Verification items for the finished model (mm, model axes). Face numbers are marked on the shaded views. A direction names the side the tool comes from. Coordinates: 2 decimals unless noted, no trailing zeros. Write each loop counter-clockwise with the first axis right and the second up, starting at its lowest first coordinate (ties: lowest second). Pieces come first, ordered by that corner, then holes. Notation, with made-up numbers: M -2.5,-4.75 L 50.5,-4.75 A20 ccw 50.5,11.25 Z; hole C -10.75,24 d7. An arc over 180 degrees is marked long. One line per item, written item: value.
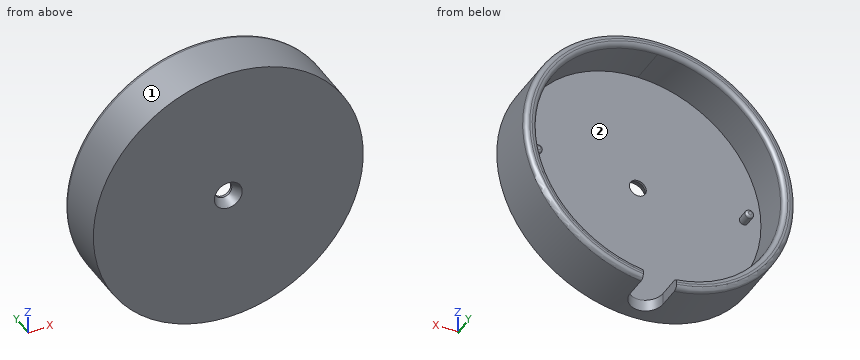
```python
from build123d import *

# Parameters (mm, degrees)
SKETCH1_R               = 56.75
BOSS_EXTRUDE3_DEPTH     = 23
SKETCH10_R              = 51.75
CUT_EXTRUDE3_DEPTH      = 18
SKETCH12_R              = 3.55
CUT_EXTRUDE4_DEPTH      = 83.250379938
SKETCH17_R              = 1.8
BOSS_EXTRUDE4_DEPTH     = 5.5
SKETCH18_R              = 1.8
BOSS_EXTRUDE5_DEPTH     = 5.5
FILLET5_R               = 1
FILLET6_R               = 1
CUT_EXTRUDE5_DEPTH      = 3
CUT_EXTRUDE5_DEPTH_BACK = 3
FILLET7_R               = 2
FILLET8_R               = 2
CHAMFER1_SIZE           = 4
CHAMFER1_SIZE2          = 2.309401077


with BuildPart() as part:
    # Sketch1 → Boss-Extrude3 (new body)
    with BuildSketch(Plane(origin=(0, 0, 0), x_dir=(1, 0, 0), z_dir=(0, 1, 0))):
        with Locations(Location((0, 0, 0), (0, 0, 270))):
            Circle(SKETCH1_R)
    extrude(amount=BOSS_EXTRUDE3_DEPTH)

    # Sketch10 → Cut-Extrude3 (cut)
    with BuildSketch(Plane(origin=(0, 23, 0), x_dir=(1, 0, 0), z_dir=(0, 1, 0))):
        with Locations(Location((0, 0, 0), (0, 0, 270))):
            Circle(SKETCH10_R)
    extrude(amount=-CUT_EXTRUDE3_DEPTH, mode=Mode.SUBTRACT)

    # Sketch12 → Cut-Extrude4 (cut, through all)
    with BuildSketch(Plane(origin=(0, 5, 0), x_dir=(1, 0, 0), z_dir=(0, 1, 0))):
        with Locations(Location((0, 0, 0), (0, 0, 270))):
            Circle(SKETCH12_R)
    extrude(amount=-CUT_EXTRUDE4_DEPTH, mode=Mode.SUBTRACT)

    # Sketch17 → Boss-Extrude4 (add)
    with BuildSketch(Plane(origin=(0, 5, 0), x_dir=(1, 0, 0), z_dir=(0, 1, 0))):
        with Locations(Location((-44.45, 0, 0), (0, 0, 270))):
            Circle(SKETCH17_R)
    extrude(amount=BOSS_EXTRUDE4_DEPTH)

    # Sketch18 → Boss-Extrude5 (add)
    with BuildSketch(Plane(origin=(0, 5, 0), x_dir=(1, 0, 0), z_dir=(0, 1, 0))):
        with Locations(Location((44.45, 0, 0), (0, 0, 270))):
            Circle(SKETCH18_R)
    extrude(amount=BOSS_EXTRUDE5_DEPTH)

    # Fillet5
    fillet5_edges = [part.edges().sort_by_distance(p)[0] for p in [
        (-44.45, 10.5, -1.8),
    ]]
    fillet(fillet5_edges, radius=FILLET5_R)

    # Fillet6
    fillet6_edges = [part.edges().sort_by_distance(p)[0] for p in [
        (44.45, 10.5, -1.8),
    ]]
    fillet(fillet6_edges, radius=FILLET6_R)

    # Sketch27 → Cut-Extrude5 (cut, two sides: drawn at the far end of the back side and taken through both)
    with BuildSketch(Plane.XY.offset(-54.25).offset(-CUT_EXTRUDE5_DEPTH_BACK)):
        with BuildLine():
            Line((7, 23), (7, 12))
            ThreePointArc((7, 12), (0, 5), (-7, 12))
            Line((-7, 12), (-7, 23))
            ThreePointArc((-7, 23), (0, 30), (7, 23))
        make_face()
    extrude(amount=CUT_EXTRUDE5_DEPTH + CUT_EXTRUDE5_DEPTH_BACK, mode=Mode.SUBTRACT)

    # Fillet7
    fillet7_edges = [part.edges().sort_by_distance(p)[0] for p in [
        (-51.630959196, 23, 3.508069632),
    ]]
    fillet(fillet7_edges, radius=FILLET7_R)

    # Fillet8
    fillet8_edges = [part.edges().sort_by_distance(p)[0] for p in [
        (-56.641553183, 23, 3.506701156),
    ]]
    fillet(fillet8_edges, radius=FILLET8_R)

    # Chamfer1
    chamfer1_edges = [part.edges().sort_by_distance(p)[0] for p in [
        (0, 0, -3.55),
    ]]
    chamfer1_side = [part.faces().sort_by_distance(p)[0] for p in [
        (0, 2.5, -3.55),
    ]]
    chamfer(chamfer1_edges, length=CHAMFER1_SIZE, length2=CHAMFER1_SIZE2, reference=chamfer1_side[0])


solid = part.part
```
Item 1: Cross-section at A-A, the plane y = 16.5. Enter the section's corners in (x, z).
The answers:
outline: M -7,-56.32 L -7,-51.27 A51.75 cw long 7,-51.27 L 7,-56.32 A56.75 ccw long Z
Item 2: Access from +Z, -Z, +X, -X, +Y, -Y to the whole of each face (thin tool, end or side, straight path). Record for the marked faces 1 and 2.
The answers:
face 1: +Y, -Y
face 2: +Y
Item 3: Go/stop test with flat-tipped pins: P1, Ø5.5, axis at y = 15.5, z = -53, coming from the -X side; P2, Ø1.3, axis at x = 44, z = 0.5, coming from the +Y side; P3, Ø1.5, axis at x = 10.5, y = 18.5, coming from the +Z side; P4, Ø5.5, axis at x = 0, z = 0, coming from the -Y side. Record where each tip stops, or that it passes through.
The answers:
P1: stops at x = -26.37
P2: stops at y = 10.5
P3: stops at z = 55.91
P4: passes through
Item 4: Scan lines: line 1 (X direction, y = 4.5, z = 0); line 2 (Y direction, x = 20.5, z = -18); line 3 (Y direction, x = -46.5, z = 29.5). Record each from-to range of solid material in increasing order.
The answers:
line 1: x = -56.75 to -3.55, 3.55 to 56.75
line 2: y = 0 to 5
line 3: y = 0 to 22.97
